Autodesk Inventor part; units mm, degrees
ref_plane "Plano de trabajo1" through (0, 0, 17.5) normal (0, 0, 1) x (1, 0, 0)
ref_plane "Plano de trabajo3" through (0, -20, 0) normal (0, 1, 0) x (-1, 0, 0)
ref_plane "YZ Plane" through (0, 0, 0) normal (1, 0, 0) x (0, 1, 0)
sketch "Boceto1" plane through (0, 0, 0) normal (0, 1, 0) x (-1, 0, 0)
  circle A0 centre (0, 0) radius 17.5
  dimension "d0" = 35
extrude "Extrusión1" add sketch "Boceto1" along normal blind 660
shell "Vaciado1" thickness 2 removed faces 2 at (-4.865, 0, -5.1831) at (-4.865, 660, -5.1831)
ref_plane "Plano de trabajo1" through (0, 0, 17.5) normal (0, 0, 1) x (1, 0, 0)
sketch "Boceto2" plane through (0, 0, 17.5) normal (0, 0, 1) x (1, 0, 0)
  line L0 (0, 714.392) -> (0, -104.9263) construction
  line L1 (-367.8002, 0) -> (437.007, 0) construction
  circle A0 centre (0, 650) radius 4
  line L2 (17.5, 660) -> (-17.5, 660)
  circle A1 centre (0, 330) radius 4
  point P0 (0, 0)
  dimension "d5" = 8
  dimension "d6" = 10
  dimension "d7" = 8
  dimension "d8" = 330
extrude "Extrusión2" cut sketch "Boceto2" against normal blind 50
ref_plane "Plano de trabajo2" through (0, 5, 0) normal (0, 1, 0) x (-1, 0, 0)
sketch "Boceto3" plane through (0, 5, 0) normal (0, 1, 0) x (-1, 0, 0)
  circle A0 centre (0, 0) radius 18.5
  dimension "d12" = 37
ref_plane "Plano de trabajo3" through (0, -20, 0) normal (0, 1, 0) x (-1, 0, 0)
sketch "Boceto4" plane through (0, -20, 0) normal (0, 1, 0) x (-1, 0, 0)
  circle A0 centre (0, 0) radius 21
  dimension "d14" = 42
loft "Solevación1" add profiles "Boceto4", "Boceto3"
Read the model definition and answer for the solid it produces. Units are mm, in the model's axes. A direction names the side the tool comes from. Round coordinates to 2 decimals unless told otherwise and drop trailing zeros. Write each loop counter-clockwise with the first axis right and the second up, starting at its lowest first coordinate (ties: lowest second). Pieces come first, ordered by that corner, then holes. Notation, with made-up numbers: M 26.5,63.5 L 69.5,63.5 A17 cw 69.5,82.5 Z; hole C 40,4.25 d5. An arc over 180 degrees is marked long. One line per item, written item: value.
Q1. Straight lines are drawn through the part: line 1 (Y direction, x = 0, z = 16); line 2 (Z direction, x = 0, y = 442.5). For each, find the intervals that lie inside material, in ascending order. Write a range as [from, to].
Data:
line 1: [-20, 326], [334, 646], [654, 660]
line 2: [-17.5, -15.5], [15.5, 17.5]
Q2. Which of the six approach directions +Z, -Z, +X, -X, +Y, -Y give full straight-line access (tool end or side, diameter ignored) to faces 4 (the flat face through (0, -20, 0)), 5 (the cylindrical face through (-14.784, 327.915, -4.656))?
Data:
face 4: +Z, -Z, +X, -X, -Y
face 5: +Y
Q3. For a pull along Z with two mould halves and no side action, classify faces 1 (the flat face through (7, 660, -14)), 2 (the conical face through (4.225, -4.897, 19.026)), 3 (the flat face through (0, 5, 0)) as +Z half, -Z half, draft (parallel to the pull), parting line (faces both ways), or undercut.
Data:
face 1: draft
face 2: parting line
face 3: undercut
Q4. Find section A-A on y = 120.5. Write down the section's boundary in (x, z), plus the area to 3 significant figures.
Data:
outline: C 0,0 d35; hole C 0,0 d31
area: 207 mm2
Q5. Flat-ended cylindrical pins translate along their axes: pin 1 Ø8 at (x, y) = (2.5, 121) entering from -Z; pin 2 Ø3 at (x, y) = (-8, 418) entering from +Z; pin 3 Ø8 at (y, z) = (363, -2) entering from -X. Find the tip coordinate at first contact, or state that the pin passes through.
Data:
pin 1: z = -17.5
pin 2: z = 16.25
pin 3: x = -17.5
